The model under review builds one solid part; all positions refer to its coordinate system, in mm. A direction names the side the tool comes from. Round coordinates to 2 decimals unless told otherwise and drop trailing zeros. Write each loop counter-clockwise with the first axis right and the second up, starting at its lowest first coordinate (ties: lowest second). Pieces come first, ordered by that corner, then holes. Notation, with made-up numbers: M -8.5,-37 L 22.5,-37 A10 cw 22.5,-28 Z; hole C 46,61 d6. An arc over 180 degrees is marked long. Write item = value, one per line. Start each with the question number.
Item 1: Take a section at C-C, the plane y = -57. Give the boundary of the cut face in (x, z), plus the area to 3 significant figures.
Item 2: Tool access review of faces 3 (the flat face through (98.5, -40.52, 28.59)), 4 (the flat face through (-40.52, 98.5, 28.59)), 5 (the flat face through (102, -1, 35)), 6 (the flat face through (76, 75, 18)), 7 (the cylindrical face through (-1.08, -104.88, 2.46)): name each direction out of +Z, -Z, +X, -X, +Y, -Y from which nothing blocks a thin tool from reaching the whole face with its end or side.
Item 3: Take a section at A-A, the plane x = -18.25. Give the boundary of the cut face in (y, z), plus the area to 3 significant figures.
Item 4: For pin 1 Ø16.5 at (x, z) = (-101, 23) entering from +Y; pin 2 Ø4.5 at (x, z) = (99.5, 18.5) entering from +Y; pin 3 Ø12 at (x, z) = (-83, 22.5) entering from -Y, all flat-tipped, find the tip position at first contact; note any pin that passes through.
Item 5: Take a section at B-B, the plane y = 0. Give the boundary of the cut face in (x, z), plus the area to 3 significant figures.
Item 6: To check wall thickness, follow line 1 along Z through (x, y) = (86, 54.5); line 2 along X through (y, z) = (15.5, 34); line 3 along Z through (x, y) = (-93.55, 18.25). State the ranges of each line that lie inside material, in increasing order.
Item 7: Take a section at D-D, the plane x = 69.5. Give the number of separate pieces and of enclosed holes in the cut face, plus the area to 3 significant figures.
Item 8: The part is to be moulded in two halves that separate along Z. For faces 1 (the flat face through (-69, -70, 5)), 2 (the flat face through (1, 90, 15)), say which applies: +Z half, -Z half, draft (parallel to the pull), parting line (faces both ways), or undercut.
from build123d import *

# Parameters (mm, degrees)
RESSALTO_EXTRUS_O1_DEPTH    = 40
CORTE_EXTRUS_O1_START       = -15
ESBO_O2_R                   = 2.7
ESBO_O2_R_2                 = 4
CORTE_EXTRUS_O1_DEPTH       = 265.198715888
CORTE_EXTRUS_O6_REACH       = 251.199
ESBO_O2_3_R                 = 4
ESBO_O2_3_R_2               = 2.7
CORTE_EXTRUS_O2_REACH       = 251.199
ESBO_O3_R                   = 4
ESBO_O3_R_2                 = 2.7
ESBO_O3_3_W                 = 74
ESBO_O3_3_H                 = 30
ESBO_O3_3_R                 = 2.7
ESBO_O3_3_R_2               = 4
CORTE_EXTRUS_O7_DEPTH       = 15
CORTE_EXTRUS_O3_REACH       = 270.559
ESBO_O4_W                   = 13
ESBO_O4_H                   = 82
CORTE_EXTRUS_O8_REACH       = 270.559
ESBO_O9_W                   = 13
ESBO_O9_H                   = 82
CORTE_EXTRUS_O9_START       = -22
CORTE_EXTRUS_O9_OUTLINE_R   = 5
CORTE_EXTRUS_O9_DEPTH       = 4
CORTE_EXTRUS_O9_START_2     = -40
CORTE_EXTRUS_O9_2_OUTLINE_R = 5
CORTE_EXTRUS_O9_2_DEPTH     = 5


# Read off the part's stored shape, not the designer's step: Corte-extrus_o9
with BuildPart() as part:
    # Esbo_o1 → Ressalto-extrus_o1 (new body)
    with BuildSketch(Plane.XY):
        Polygon((110, 45.563491861), (45.563491861, 110), (-45.563491861, 110), (-110, 45.563491861), (-110, -45.563491861), (-45.563491861, -110), (45.563491861, -110), (110, -45.563491861), align=None)
        Polygon((90, 37.279220614), (37.279220614, 90), (-37.279220614, 90), (-90, 37.279220614), (-90, -37.279220614), (-37.279220614, -90), (37.279220614, -90), (90, -37.279220614), align=None, mode=Mode.SUBTRACT)
    extrude(amount=RESSALTO_EXTRUS_O1_DEPTH)

    # Esbo_o2 → Corte-extrus_o1 (cut)
    with BuildSketch(Plane(origin=(110, 0, 0), x_dir=(0, 0, -1), z_dir=(1, 0, 0)).offset(CORTE_EXTRUS_O1_START)):
        Polygon((-35, 37), (-5, 37), (-5, -37.017144549), (-5, -37), (-35, -37), (-35, -37.017144549), align=None)
        with Locations(Location((-20, -18.25, 0), (0, 0, 270))):
            Circle(ESBO_O2_R, mode=Mode.SUBTRACT)
        with Locations(Location((-20, 18.25, 0), (0, 0, 270))):
            Circle(ESBO_O2_R, mode=Mode.SUBTRACT)
        with Locations(Location((-20, 0, 0), (0, 0, 270))):
            Circle(ESBO_O2_R_2, mode=Mode.SUBTRACT)
    corte_extrus_o1 = extrude(amount=CORTE_EXTRUS_O1_DEPTH, mode=Mode.SUBTRACT)

    # Esbo_o2_3 → Corte-extrus_o6 (cut, up to next)
    with BuildSketch(Plane(origin=(110, 0, 0), x_dir=(0, 0, -1), z_dir=(1, 0, 0)), mode=Mode.PRIVATE) as corte_extrus_o6_sk1:
        with Locations(Location((-20, 0, 0), (0, 0, 90))):
            Circle(ESBO_O2_3_R)
    corte_extrus_o6_tool1 = extrude(corte_extrus_o6_sk1.sketch, amount=-CORTE_EXTRUS_O6_REACH, mode=Mode.PRIVATE) & part.part
    # Esbo_o2_3 → Corte-extrus_o6 (cut, up to next)
    with BuildSketch(Plane(origin=(110, 0, 0), x_dir=(0, 0, -1), z_dir=(1, 0, 0)), mode=Mode.PRIVATE) as corte_extrus_o6_sk2:
        with Locations(Location((-20, -18.25, 0), (0, 0, 90))):
            Circle(ESBO_O2_3_R_2)
    corte_extrus_o6_tool2 = extrude(corte_extrus_o6_sk2.sketch, amount=-CORTE_EXTRUS_O6_REACH, mode=Mode.PRIVATE) & part.part
    # Esbo_o2_3 → Corte-extrus_o6 (cut, up to next)
    with BuildSketch(Plane(origin=(110, 0, 0), x_dir=(0, 0, -1), z_dir=(1, 0, 0)), mode=Mode.PRIVATE) as corte_extrus_o6_sk3:
        with Locations(Location((-20, 18.25, 0), (0, 0, 90))):
            Circle(ESBO_O2_3_R_2)
    corte_extrus_o6_tool3 = extrude(corte_extrus_o6_sk3.sketch, amount=-CORTE_EXTRUS_O6_REACH, mode=Mode.PRIVATE) & part.part
    corte_extrus_o6_1 = corte_extrus_o6_tool1.solids().sort_by_distance((110, 0, 20))[0]
    add(corte_extrus_o6_1, mode=Mode.SUBTRACT)
    corte_extrus_o6_2 = corte_extrus_o6_tool2.solids().sort_by_distance((110, -18.25, 20))[0]
    add(corte_extrus_o6_2, mode=Mode.SUBTRACT)
    corte_extrus_o6_3 = corte_extrus_o6_tool3.solids().sort_by_distance((110, 18.25, 20))[0]
    add(corte_extrus_o6_3, mode=Mode.SUBTRACT)
    corte_extrus_o6 = corte_extrus_o6_1 + corte_extrus_o6_2 + corte_extrus_o6_3  # Corte-extrus_o6 as one shape, for the pattern or mirror that repeats it

    # Esbo_o3 → Corte-extrus_o2 (cut, up to next)
    with BuildSketch(Plane(origin=(0, 110, 0), x_dir=(1, 0, 0), z_dir=(0, 1, 0)), mode=Mode.PRIVATE) as corte_extrus_o2_sk1:
        with Locations(Location((0, -20, 0), (0, 0, 180))):
            Circle(ESBO_O3_R)
    corte_extrus_o2_tool1 = extrude(corte_extrus_o2_sk1.sketch, amount=-CORTE_EXTRUS_O2_REACH, mode=Mode.PRIVATE) & part.part
    # Esbo_o3 → Corte-extrus_o2 (cut, up to next)
    with BuildSketch(Plane(origin=(0, 110, 0), x_dir=(1, 0, 0), z_dir=(0, 1, 0)), mode=Mode.PRIVATE) as corte_extrus_o2_sk2:
        with Locations(Location((18.25, -20, 0), (0, 0, 180))):
            Circle(ESBO_O3_R_2)
    corte_extrus_o2_tool2 = extrude(corte_extrus_o2_sk2.sketch, amount=-CORTE_EXTRUS_O2_REACH, mode=Mode.PRIVATE) & part.part
    # Esbo_o3 → Corte-extrus_o2 (cut, up to next)
    with BuildSketch(Plane(origin=(0, 110, 0), x_dir=(1, 0, 0), z_dir=(0, 1, 0)), mode=Mode.PRIVATE) as corte_extrus_o2_sk3:
        with Locations(Location((-18.25, -20, 0), (0, 0, 180))):
            Circle(ESBO_O3_R_2)
    corte_extrus_o2_tool3 = extrude(corte_extrus_o2_sk3.sketch, amount=-CORTE_EXTRUS_O2_REACH, mode=Mode.PRIVATE) & part.part
    corte_extrus_o2_1 = corte_extrus_o2_tool1.solids().sort_by_distance((0, 110, 20))[0]
    add(corte_extrus_o2_1, mode=Mode.SUBTRACT)
    corte_extrus_o2_2 = corte_extrus_o2_tool2.solids().sort_by_distance((18.25, 110, 20))[0]
    add(corte_extrus_o2_2, mode=Mode.SUBTRACT)
    corte_extrus_o2_3 = corte_extrus_o2_tool3.solids().sort_by_distance((-18.25, 110, 20))[0]
    add(corte_extrus_o2_3, mode=Mode.SUBTRACT)
    corte_extrus_o2 = corte_extrus_o2_1 + corte_extrus_o2_2 + corte_extrus_o2_3  # Corte-extrus_o2 as one shape, for the pattern or mirror that repeats it

    # Espelhar1: Corte-extrus_o1, Corte-extrus_o6 across plane
    add(corte_extrus_o1.mirror(Plane(origin=(0, 0, 0), x_dir=(0, 0, 1), z_dir=(1, 0, 0))), mode=Mode.SUBTRACT)
    add(corte_extrus_o6.mirror(Plane(origin=(0, 0, 0), x_dir=(0, 0, 1), z_dir=(1, 0, 0))), mode=Mode.SUBTRACT)

    # Esbo_o3_3 → Corte-extrus_o7 (cut)
    with BuildSketch(Plane(origin=(0, 110, 0), x_dir=(1, 0, 0), z_dir=(0, 1, 0))):
        with Locations((0, -20)):
            Rectangle(ESBO_O3_3_W, ESBO_O3_3_H)
        with Locations(Location((-18.25, -20, 0), (0, 0, 180))):
            Circle(ESBO_O3_3_R, mode=Mode.SUBTRACT)
        with Locations(Location((0, -20, 0), (0, 0, 180))):
            Circle(ESBO_O3_3_R_2, mode=Mode.SUBTRACT)
        with Locations(Location((18.25, -20, 0), (0, 0, 180))):
            Circle(ESBO_O3_3_R, mode=Mode.SUBTRACT)
    corte_extrus_o7 = extrude(amount=-CORTE_EXTRUS_O7_DEPTH, mode=Mode.SUBTRACT)

    # Espelhar2: Corte-extrus_o2, Corte-extrus_o7 across plane
    add(corte_extrus_o2.mirror(Plane.ZX), mode=Mode.SUBTRACT)
    add(corte_extrus_o7.mirror(Plane.ZX), mode=Mode.SUBTRACT)

    # Esbo_o4 → Corte-extrus_o3 (cut, up to next)
    with BuildSketch(Plane(origin=(77.781745931, 77.781745931, 0), x_dir=(0, 0, -1), z_dir=(0.707106781186547, 0.7071067811865481, 0)), mode=Mode.PRIVATE) as corte_extrus_o3_sk1:
        with Locations((-11.5, 0)):
            Rectangle(ESBO_O4_W, ESBO_O4_H)
    corte_extrus_o3_tool1 = extrude(corte_extrus_o3_sk1.sketch, amount=-CORTE_EXTRUS_O3_REACH, mode=Mode.PRIVATE) & part.part
    # Esbo_o4 → Corte-extrus_o3 (cut, up to next)
    with BuildSketch(Plane(origin=(77.781745931, 77.781745931, 0), x_dir=(0, 0, -1), z_dir=(0.707106781186547, 0.7071067811865481, 0)), mode=Mode.PRIVATE) as corte_extrus_o3_sk2:
        with Locations((-28.5, 0)):
            Rectangle(ESBO_O4_W, ESBO_O4_H)
    corte_extrus_o3_tool2 = extrude(corte_extrus_o3_sk2.sketch, amount=-CORTE_EXTRUS_O3_REACH, mode=Mode.PRIVATE) & part.part
    corte_extrus_o3_1 = corte_extrus_o3_tool1.solids().sort_by_distance((77.781746, 77.781746, 11.5))[0]
    add(corte_extrus_o3_1, mode=Mode.SUBTRACT)
    corte_extrus_o3_2 = corte_extrus_o3_tool2.solids().sort_by_distance((77.781746, 77.781746, 28.5))[0]
    add(corte_extrus_o3_2, mode=Mode.SUBTRACT)
    corte_extrus_o3 = corte_extrus_o3_1 + corte_extrus_o3_2  # Corte-extrus_o3 as one shape, for the pattern or mirror that repeats it

    # Espelhar3: Corte-extrus_o3 across plane
    add(corte_extrus_o3.mirror(Plane(origin=(0, 0, 0), x_dir=(0, 0, 1), z_dir=(0.7071067811865475, 0.7071067811865477, 0))), mode=Mode.SUBTRACT)

    # Esbo_o9 → Corte-extrus_o8 (cut, up to next)
    with BuildSketch(Plane(origin=(77.781745931, -77.781745931, 0), x_dir=(0, 0, -1), z_dir=(0.7071067811865479, -0.7071067811865471, 0)), mode=Mode.PRIVATE) as corte_extrus_o8_sk1:
        with Locations((-11.5, 0)):
            Rectangle(ESBO_O9_W, ESBO_O9_H)
    corte_extrus_o8_tool1 = extrude(corte_extrus_o8_sk1.sketch, amount=-CORTE_EXTRUS_O8_REACH, mode=Mode.PRIVATE) & part.part
    # Esbo_o9 → Corte-extrus_o8 (cut, up to next)
    with BuildSketch(Plane(origin=(77.781745931, -77.781745931, 0), x_dir=(0, 0, -1), z_dir=(0.7071067811865479, -0.7071067811865471, 0)), mode=Mode.PRIVATE) as corte_extrus_o8_sk2:
        with Locations((-28.5, 0)):
            Rectangle(ESBO_O9_W, ESBO_O9_H)
    corte_extrus_o8_tool2 = extrude(corte_extrus_o8_sk2.sketch, amount=-CORTE_EXTRUS_O8_REACH, mode=Mode.PRIVATE) & part.part
    corte_extrus_o8_1 = corte_extrus_o8_tool1.solids().sort_by_distance((77.781746, -77.781746, 11.5))[0]
    add(corte_extrus_o8_1, mode=Mode.SUBTRACT)
    corte_extrus_o8_2 = corte_extrus_o8_tool2.solids().sort_by_distance((77.781746, -77.781746, 28.5))[0]
    add(corte_extrus_o8_2, mode=Mode.SUBTRACT)
    corte_extrus_o8 = corte_extrus_o8_1 + corte_extrus_o8_2  # Corte-extrus_o8 as one shape, for the pattern or mirror that repeats it

    # Espelhar4: Corte-extrus_o8 across plane
    add(corte_extrus_o8.mirror(Plane(origin=(0, 0, 0), x_dir=(0, 0, 1), z_dir=(0.7071067811865475, -0.7071067811865477, 0))), mode=Mode.SUBTRACT)

    # Corte-extrus_o9 outline → Corte-extrus_o9 (cut)
    with BuildSketch(Plane.XY.offset(40).offset(CORTE_EXTRUS_O9_START)):
        with Locations((-70.710678119, 70.710678119)):
            Circle(CORTE_EXTRUS_O9_OUTLINE_R)
        with Locations((70.710678119, -70.710678119)):
            Circle(CORTE_EXTRUS_O9_OUTLINE_R)
        with Locations((-70.710678119, -70.710678119)):
            Circle(CORTE_EXTRUS_O9_OUTLINE_R)
        with Locations((70.710678119, 70.710678119)):
            Circle(CORTE_EXTRUS_O9_OUTLINE_R)
    extrude(amount=CORTE_EXTRUS_O9_DEPTH, mode=Mode.SUBTRACT)

    # Corte-extrus_o9 2 outline → Corte-extrus_o9 2 (cut)
    with BuildSketch(Plane.XY.offset(40).offset(CORTE_EXTRUS_O9_START_2)):
        with Locations((0, -100)):
            Circle(CORTE_EXTRUS_O9_2_OUTLINE_R)
    extrude(amount=CORTE_EXTRUS_O9_2_DEPTH, mode=Mode.SUBTRACT)


solid = part.part
Response values:
q1.outline = M -98.56,0 L -70.28,0 L -70.28,5 L -98.56,5 Z; M -98.56,18 L -70.28,18 L -70.28,22 L -98.56,22 Z; M -98.56,35 L -70.28,35 L -70.28,40 L -98.56,40 Z; M 70.28,0 L 98.56,0 L 98.56,5 L 70.28,5 Z; M 70.28,18 L 98.56,18 L 98.56,22 L 70.28,22 Z; M 70.28,35 L 98.56,35 L 98.56,40 L 70.28,40 Z
q1.area = 792 mm2
q2.face_3 = -Y
q2.face_4 = -X
q2.face_5 = +X
q2.face_6 = none
q2.face_7 = -Z
q3.outline = M -110,0 L -90,0 L -90,17.3 L -95,17.3 L -95,5 L -110,5 Z; M -110,35 L -95,35 L -95,22.7 L -90,22.7 L -90,40 L -110,40 Z; M 90,0 L 110,0 L 110,5 L 95,5 L 95,17.3 L 90,17.3 Z; M 90,22.7 L 95,22.7 L 95,35 L 110,35 L 110,40 L 90,40 Z
q3.area = 646 mm2
q4.pin_1 = 62.75
q4.pin_2 = 58.31
q4.pin_3 = -78.54
q5.outline = M -110,0 L -90,0 L -90,16 L -95,16 L -95,5 L -110,5 Z; M -110,35 L -95,35 L -95,24 L -90,24 L -90,40 L -110,40 Z; M 90,0 L 110,0 L 110,5 L 95,5 L 95,16 L 90,16 Z; M 90,24 L 95,24 L 95,35 L 110,35 L 110,40 L 90,40 Z
q5.area = 620 mm2
q6.line_1 = 0 to 5, 18 to 22, 35 to 40
q6.line_2 = -95 to -90, 90 to 95
q6.line_3 = 0 to 17.3, 22.7 to 40
q7.separate_pieces = 8
q7.enclosed_holes = 0
q7.area = 714 mm2
q8.face_1 = undercut
q8.face_2 = draft
